```python
from build123d import *

# Parameters (mm, degrees)
F0_W     = 180
F0_H     = 75
F0_R     = 1.6
F0_W_2   = 10
F0_H_2   = 8
F0_R_2   = 3
F0_R_3   = 3.9624
F1_DEPTH = 6
F2_R     = 5


with BuildPart() as f1:
    # F0 (on Top) → F1 (new body)
    with BuildSketch(Plane.XY):
        Rectangle(F0_W, F0_H)
        with BuildLine():
            ThreePointArc((-26.0376, -9.5475), (-32.80184, -12.34934), (-30, -5.5851))
            ThreePointArc((-30, -5.5851), (-27.19816, -6.74566), (-26.0376, -9.5475))
        make_face(mode=Mode.SUBTRACT)
        with Locations((10, -22.5)):
            Circle(F0_R, mode=Mode.SUBTRACT)
        with Locations((49.7, -1.06)):
            Circle(F0_R, mode=Mode.SUBTRACT)
        with Locations((-55, 0)):
            Rectangle(F0_W_2, F0_H_2, mode=Mode.SUBTRACT)
        with BuildLine():
            ThreePointArc((-30, 5.5401), (-32.80184, 12.30434), (-26.0376, 9.5025))
            ThreePointArc((-26.0376, 9.5025), (-27.19816, 6.70066), (-30, 5.5401))
        make_face(mode=Mode.SUBTRACT)
        with Locations((0, 17.5)):
            Circle(F0_R_2, mode=Mode.SUBTRACT)
        with Locations((40, 17.5)):
            Circle(F0_R_3, mode=Mode.SUBTRACT)
        with Locations((59.05, 17.5)):
            Circle(F0_R_3, mode=Mode.SUBTRACT)
    extrude(amount=F1_DEPTH)

    # F2
    f2_edges = [f1.edges().sort_by_distance(p)[0] for p in [
        (-90, 37.5, 3),
        (90, 37.5, 3),
        (90, -37.5, 3),
        (-90, -37.5, 3),
    ]]
    fillet(f2_edges, radius=F2_R)


solid = f1.part
```
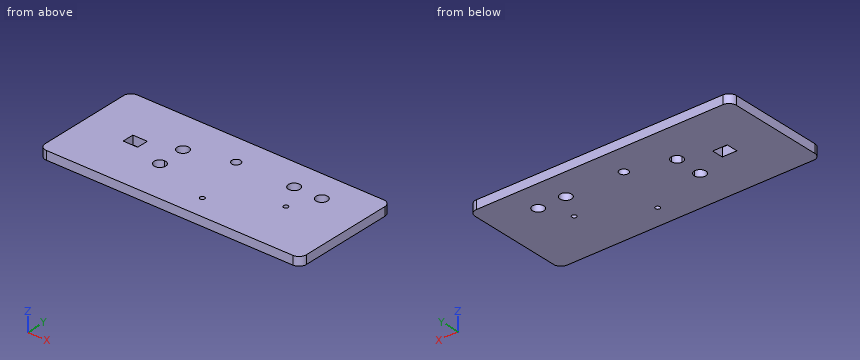
Input: part model. Units: mm. Frame: model coordinates. Round coordinates to 2 decimals unless told otherwise and drop trailing zeros. Write each loop counter-clockwise with the first axis right and the second up, starting at its lowest first coordinate (ties: lowest second). Pieces come first, ordered by that corner, then holes. Notation, with made-up numbers: M 53,10.5 L 82,10.5 A16 ccw 82,32.5 Z; hole C 13.25,26 d7. An arc over 180 degrees is marked long. Write each question's results on one line, items separated by ' | '.
Q1. Section query B-B (x = 49.7). Return loops of the section in (y, z), and give its area (3 significant figures).
Results:
outline: M -37.5,0 L -2.66,0 L -2.66,6 L -37.5,6 Z; M 0.54,0 L 37.5,0 L 37.5,6 L 0.54,6 Z | area: 431 mm^2
Q2. Section query D-D (y = -22.5). Return loops of the section in (x, z).
Results:
outline: M -90,0 L 8.4,0 L 8.4,6 L -90,6 Z; M 11.6,0 L 90,0 L 90,6 L 11.6,6 Z
Q3. Line query: line 1 along Y through (x, z) = (59.05, 3.35); line 2 along X through (y, z) = (1, 1.7); line 3 along Y through (x, z) = (-30, 3.15). Output: solid intervals per line, ascending.
Results:
line 1: y = -37.5 to 13.54, 21.46 to 37.5 | line 2: x = -90 to -60, -50 to 90 | line 3: y = -37.5 to -13.51, -5.59 to 5.54, 13.46 to 37.5
Q4. Section query C-C (z = 1.5). State how many separate pieces and enclosed holes the cut face has, and give its area (3 significant figures).
Results:
separate pieces: 1 | enclosed holes: 8 | area: 13,200 mm^2
Q5. Section query A-A (y = 17.5). Return loops of the section in (x, z), and give its area (3 significant figures).
Results:
outline: M -90,0 L -3,0 L -3,6 L -90,6 Z; M 3,0 L 36.04,0 L 36.04,6 L 3,6 Z; M 43.96,0 L 55.09,0 L 55.09,6 L 43.96,6 Z; M 63.01,0 L 90,0 L 90,6 L 63.01,6 Z | area: 949 mm^2
